```python
from build123d import *

# Parameters (mm, degrees)
SKETCH_1_W          = 8
SKETCH_1_H          = 1.25
CHAMFER_1_SIZE      = 0.5
CUT_EXTRUDE_1_DEPTH = 1


with BuildPart() as part:
    # Эскиз1 → Повернуть1 (revolve)
    with BuildSketch(Plane.XY):
        with Locations((4, 1.875)):
            Rectangle(SKETCH_1_W, SKETCH_1_H)
    revolve(axis=Axis((0, 0, 0), (1, 0, 0)))

    # Эскиз2 → Отверстие обработанное метчиком M31 (revolve, cut)
    with BuildSketch(Plane(origin=(8, 0, 0), x_dir=(0, 0, -1), z_dir=(0, 1, 0))):
        Polygon((0, 0), (0, 8), (1.6, 8), (1.25, 7.754927362), (1.25, 0.245072638), (1.6, 0), align=None)
    revolve(axis=Axis((14.35, 0, 0), (-1, 0, 0)), mode=Mode.SUBTRACT)

    # Фаска1
    chamfer_1_edges = [part.edges().sort_by_distance(p)[0] for p in [
        (8, -2.5, 0),
    ]]
    chamfer(chamfer_1_edges, length=CHAMFER_1_SIZE)

    # Эскиз4 → Вырез-Вытянуть1 (cut)
    with BuildSketch(Plane.ZY):
        with BuildLine():
            ThreePointArc((1.5, 2), (0, 2.5), (-1.5, 2))
            Line((-1.5, 2), (1.5, 2))
        make_face()
        with BuildLine():
            Line((1.5, -2), (-1.5, -2))
            ThreePointArc((-1.5, -2), (0, -2.5), (1.5, -2))
        make_face()
    extrude(amount=-CUT_EXTRUDE_1_DEPTH, mode=Mode.SUBTRACT)


solid = part.part
```
Work out the finished part from the listing and answer in its coordinate system (mm). A direction names the side the tool comes from. Coordinates: 2 decimals unless noted, no trailing zeros. Loops run counter-clockwise (first coordinate to the right, second up) from the corner with the lowest first, then second, coordinate; pieces in that order, holes last. Notation, with made-up numbers: M 73,76.25 L 116,76.25 A29 ccw 116,107.25 Z; hole C 25.5,74 d3. An arc over 180 degrees is marked long. Use CSV: the item, a comma, the result in double quotes. Start each with the question number.
(1) Find section B-B, the plane y = 0. Give the vertices of the cut face in (x, z).
(2) For a pull along Y with two mould halves and no side action, classify faces 3 (the face through (4.053, 1.155, -0.479)), 4 (the face through (0.5, 2, 0)), 5 (the face through (3.8, -2.5, 0.1)) as +Y half, -Y half, draft (parallel to the pull), parting line (faces both ways), or undercut.
(3) Find section A-A, the plane z = 0. Give the vertices of the cut face in (x, y).
(4) Find section C-C, the plane x = 1.75. Give the vertices of the cut face in (y, z).
(5) Consider line 1 (Z direction, x = 6, y = 0); line 2 (Y direction, x = 4, z = 0.65). Determine where each line is inside the solid, lowest interval first.
(6) For faces 1 (the face through (0, 0, 2)), 2 (the face through (0.5, -2, 0)), determine the directions among +Z, -Z, +X, -X, +Y, -Y from which every point of the face is accessible in a straight line to the end or side of a thin tool.
Recorded:
1,outline,"M 0,-2.5 L 7.5,-2.5 L 8,-2 L 8,-1.6 L 7.75,-1.25 L 0.25,-1.25 L 0,-1.6 Z; M 0,1.6 L 0.25,1.25 L 7.75,1.25 L 8,1.6 L 8,2 L 7.5,2.5 L 0,2.5 Z"
2,face 3,"undercut"
2,face 4,"+Y half"
2,face 5,"parting line"
3,outline,"M 0,-2 L 1,-2 L 1,-2.5 L 7.5,-2.5 L 8,-2 L 8,-1.6 L 7.75,-1.25 L 0.25,-1.25 L 0,-1.6 Z; M 0,1.6 L 0.25,1.25 L 7.75,1.25 L 8,1.6 L 8,2 L 7.5,2.5 L 1,2.5 L 1,2 L 0,2 Z"
4,outline,"C 0,0 d5; hole C 0,0 d2.5"
5,line 1,"z = -2.5 to -1.25, 1.25 to 2.5"
5,line 2,"y = -2.41 to -1.07, 1.07 to 2.41"
6,face 1,"+Z, -Z, -X, +Y, -Y"
6,face 2,"+Z, -Z, -X, -Y"
